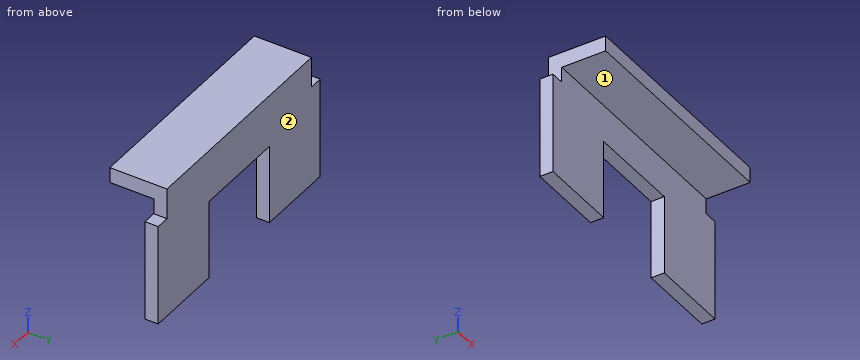
from build123d import *

# Parameters (mm, degrees)
BOSS_EXTRUDE1_DEPTH = 3
SKETCH3_W           = 51.3
SKETCH3_H           = 3.5
BOSS_EXTRUDE2_DEPTH = 10


with BuildPart() as part:
    # Sketch2 → Boss-Extrude1 (new body)
    with BuildSketch(Plane(origin=(0, 0, 0), x_dir=(1, 0, 0), z_dir=(0, 1, 0))):
        Polygon((-25.65, 0), (0, 0), (0, 12), (-10.75, 12), (-10.75, 30), (-28.75, 30), (-28.75, 7), (-25.65, 7), align=None)
        Polygon((0, 0), (25.65, 0), (25.65, 7), (28.75, 7), (28.75, 30), (10.75, 30), (10.75, 12), (0, 12), align=None)
    extrude(amount=BOSS_EXTRUDE1_DEPTH)

    # Sketch3 → Boss-Extrude2 (add)
    with BuildSketch(Plane.XZ):
        with Locations((0, -1.75)):
            Rectangle(SKETCH3_W, SKETCH3_H)
    extrude(amount=BOSS_EXTRUDE2_DEPTH)


solid = part.part
CAD build for the part. Positions are in the model's coordinates, mm. Face numbers are marked on the shaded views. A direction names the side the tool comes from. Give positions to 0.01 mm unless a question says otherwise; leave off trailing zeros. Loops run counter-clockwise (first coordinate to the right, second up) from the corner with the lowest first, then second, coordinate; pieces in that order, holes last. Notation, with made-up numbers: M 47.5,63.5 L 72.5,63.5 A12 ccw 72.5,74.5 Z; hole C 2,6.5 d2. An arc over 180 degrees is marked long. Write each question's results on one line, items separated by ' | '.
Q1. Band-saw the part on A-A on z = -17. Write the cut outline in (x, y).
Geometry check:
outline: M -28.75,0 L -10.75,0 L -10.75,3 L -28.75,3 Z; M 10.75,0 L 28.75,0 L 28.75,3 L 10.75,3 Z
Q2. Which spindle directions (+Z, -Z, +X, -X, +Y, -Y) get a long thin tool onto all of the face, cutting with end or side? Do the marked faces 1 and 2. Say none if no direction does.
Geometry check:
face 1: -Z, +X, -X, -Y | face 2: +Z, -Z, +X, -X, +Y
Q3. Band-saw the part on C-C on x = -12.5. Write the cut outline in (y, z).
Geometry check:
outline: M -10,-3.5 L 0,-3.5 L 0,-30 L 3,-30 L 3,0 L -10,0 Z
Q4. Band-saw the part on D-D on y = -8.5. Write the cut outline in (x, z).
Geometry check:
outline: M -25.65,-3.5 L 25.65,-3.5 L 25.65,0 L -25.65,0 Z
Q5. Band-saw the part on B-B on y = 1.5. Write the cut outline in (x, z).
Geometry check:
outline: M -28.75,-30 L -10.75,-30 L -10.75,-12 L 10.75,-12 L 10.75,-30 L 28.75,-30 L 28.75,-7 L 25.65,-7 L 25.65,0 L -25.65,0 L -25.65,-7 L -28.75,-7 Z
Q6. Flat gauge pins, fed straight in: P1, Ø0.9, axis at x = 26.5, y = 2, coming from the +Z side; P2, Ø3.5, axis at y = -1, z = -4.5, coming from the -X side; P3, Ø8, axis at x = 13.5, z = -18.5, coming from the -Y side. Where does each tip first touch, or does it go through?
Geometry check:
P1: stops at z = -7 | P2: stops at x = -25.65 | P3: stops at y = 0
Q7. Probe probe 1 along X at (y, z) = (1.25, -26.25); probe 2 along Z at (x, y) = (8, 2); probe 3 along Y at (x, z) = (-11, -5). List the from-to ranges inside material, lowest first.
Geometry check:
probe 1: x = -28.75 to -10.75, 10.75 to 28.75 | probe 2: z = -12 to 0 | probe 3: y = 0 to 3
